Verification items for this drawing (mm, ordinates from the low corner). Round coordinates to 2 decimals unless told otherwise and drop trailing zeros. Loops run counter-clockwise (first coordinate to the right, second up) from the corner with the lowest first, then second, coordinate; pieces in that order, holes last. Notation, with made-up numbers: (69.5, 89.5) -> (122.5, 89.5) arc R23 ccw to (122.5, 122.5) -> close; hole circle Ø11 at (58.5, 23.25). An arc over 180 degrees is marked (long way). One line per question, with ' | ' between items.
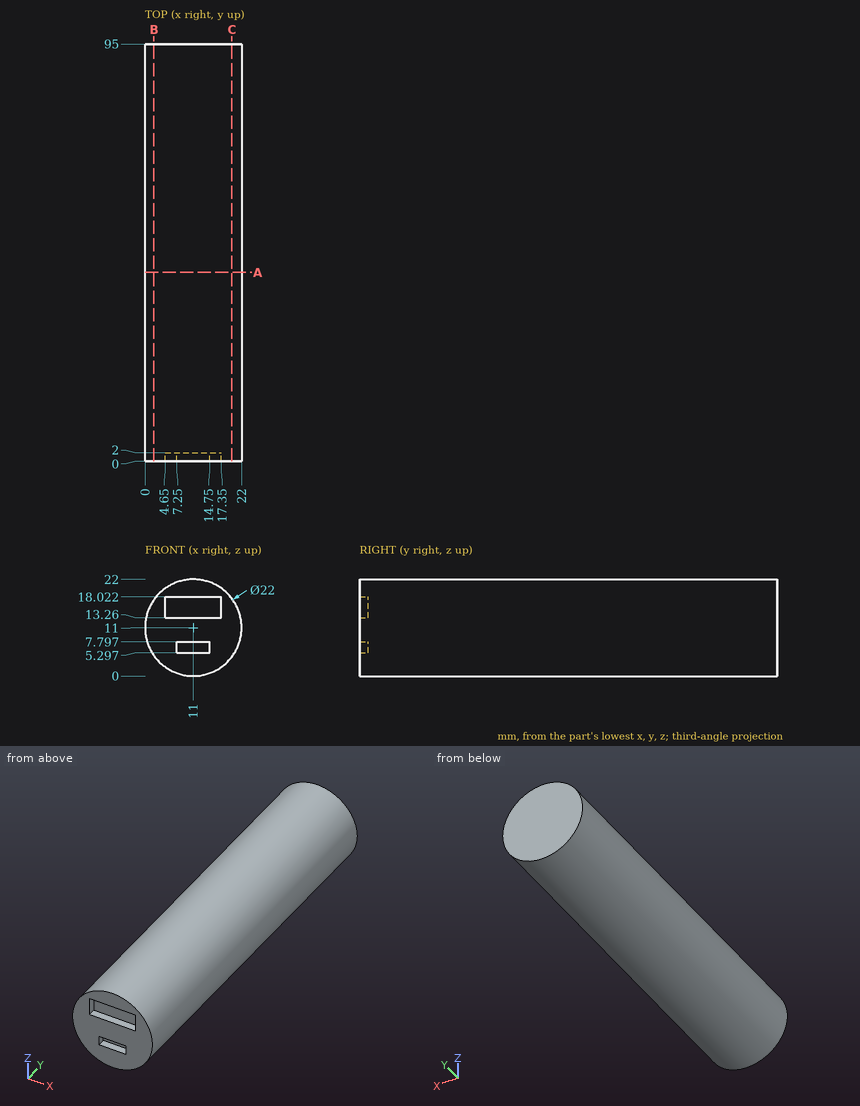
(1) Sectioned sample at A-A, the plane y = 43. Record the cut outline in (x, z).
Answer:
outline: circle Ø22 at (11, 11)
(2) Go/stop test with flat-tipped pins: pin 1 (0.6 mm diameter, centred on y = 1.5, z = 16.5, fed in from +X); pin 2 (1.6 mm diameter, centred on y = 0.5, z = 16, fed in from -X); pin 3 (4 mm diameter, centred on x = 19, y = 60.5, fed in from +Z). Record where each tip stops, or that it passes through.
Answer:
pin 1: stops at x = 20.69 | pin 2: stops at x = 0.83 | pin 3: stops at z = 20.22
(3) Scan lines: probe 1 along Y at (x, z) = (7.25, 17.25); probe 2 along X at (y, z) = (15.5, 11.5); probe 3 along Z at (x, y) = (3.5, 75.5) (1 decimal). Record each from-to range of solid material in increasing order.
Answer:
probe 1: y = 2 to 95 | probe 2: x = 0.01 to 21.99 | probe 3: z = 3 to 19
(4) Sectioned sample at B-B, the plane x = 2. Record the cut outline in (y, z) (1 decimal).
Answer:
outline: (0, 4.7) -> (95, 4.7) -> (95, 17.3) -> (0, 17.3) -> close
(5) Sectioned sample at C-C, the plane x = 19.75. Record the cut outline in (y, z).
Answer:
outline: (0, 4.33) -> (95, 4.33) -> (95, 17.67) -> (0, 17.67) -> close
